Part model, mm, in its own coordinate system. Face numbers are marked on the shaded views. Coordinates: 2 decimals unless noted, no trailing zeros. Order: outer loops, then holes, each group sorted by start corner. A loop starts at its lowest first (then second) coordinate and runs counter-clockwise, first axis right, second up. Notation, with made-up numbers: (68.5, 56) - (120.5, 56) arc R38 ccw to (120.5, 94) - close; hole circle Ø7 at (11.5, 53.5). An arc over 180 degrees is marked (long way). Use a Markdown table: item, result. Add a question column.
1) Drop flat-ended pins along their axis: P1, Ø1.5, axis at x = 94.5, y = 57, coming from the +Z side; P2, Ø3, axis at x = -96.5, z = 127.5, coming from the +Y side; P3, Ø1.5, axis at x = 26, z = 43, coming from the +Y side. Give the stop position or say it passes through.
2) Saw through at B-B on y = 15. Count the separate pieces of the cut face and the enclosed holes in it, then the cut area to 3 significant figures.
3) Wall check: L1, parallel to X at y = -2.5, z = 27.5; L2, parallel to Z at x = -96, y = -2; L3, parallel to Z at x = -96.5, y = -2.05. Give the ranges that are in metal, low to high. Write a range as [from, to].
4) Saw through at A-A on z = 9. List the corners of the cut face in (x, y), then the cut area to 3 significant figures.
5) Two-plate mould, pull along X, no slides. Class the marked faces 1 and 2: +X half, -X half, draft (parallel to the pull), parting line (faces both ways), or undercut.
6) Saw through at C-C on x = 33.5. List the corners of the cut face in (y, z), then the cut area to 3 significant figures.
```python
from build123d import *

# Parameters (mm, degrees)
BOSS_EXTRUDE1_DEPTH      = 160
BOSS_EXTRUDE1_2_DEPTH    = 160
LPATTERN1_COUNT          = 3
LPATTERN1_PITCH          = 55
SKETCH2_W                = 201
SKETCH2_H                = 143
BOSS_EXTRUDE2_DEPTH      = 5
BOSS_EXTRUDE3_DEPTH      = 8
M3_CLEARANCE_HOLE1_D     = 3.4
M3_CLEARANCE_HOLE1_DEPTH = 5


with BuildPart() as part:
    # Sketch1 → Boss-Extrude1 (new body)
    with BuildSketch(Plane(origin=(0, 0, 0), x_dir=(1, 0, 0), z_dir=(0, 1, 0))):
        Polygon((-100.5, 5.5), (-92.5, 5.5), (-92.5, 2.5), (-97.5, 2.5), (-97.5, -2.5), (-92.5, -2.5), (-92.5, -5.5), (-100.5, -5.5), align=None)
    boss_extrude1 = extrude(amount=BOSS_EXTRUDE1_DEPTH)



with BuildPart() as body_2:
    # Sketch1 → Boss-Extrude1 2 (new body)
    with BuildSketch(Plane(origin=(0, 0, 0), x_dir=(1, 0, 0), z_dir=(0, 1, 0))):
        Polygon((100.5, -5.5), (100.5, 5.5), (92.5, 5.5), (92.5, 2.5), (97.5, 2.5), (97.5, -2.5), (92.5, -2.5), (92.5, -5.5), align=None)
    boss_extrude1_2 = extrude(amount=BOSS_EXTRUDE1_2_DEPTH)


with BuildPart() as lpattern1_1:
    # LPattern1: pattern copy
    add(boss_extrude1.moved(Location(Vector(0, 0, 1) * (1 * LPATTERN1_PITCH))))


with BuildPart() as lpattern1_2:
    # LPattern1: pattern copy
    add(boss_extrude1.moved(Location(Vector(0, 0, 1) * (2 * LPATTERN1_PITCH))))


with BuildPart() as lpattern1_3:
    # LPattern1: pattern copy
    add(boss_extrude1_2.moved(Location(Vector(0, 0, 1) * (1 * LPATTERN1_PITCH))))


with BuildPart() as lpattern1_4:
    # LPattern1: pattern copy
    add(boss_extrude1_2.moved(Location(Vector(0, 0, 1) * (2 * LPATTERN1_PITCH))))


with BuildPart() as part_1:
    add(part.part)

    add(body_2.part)  # Boss-Extrude2 merges body 2

    add(lpattern1_1.part)  # Boss-Extrude2 merges LPattern1_1

    add(lpattern1_2.part)  # Boss-Extrude2 merges LPattern1_2

    add(lpattern1_3.part)  # Boss-Extrude2 merges LPattern1_3

    add(lpattern1_4.part)  # Boss-Extrude2 merges LPattern1_4
    # Sketch2 → Boss-Extrude2 (add)
    with BuildSketch(Plane.XZ):
        with Locations((0, 66)):
            Rectangle(SKETCH2_W, SKETCH2_H)
    extrude(amount=BOSS_EXTRUDE2_DEPTH)

    # Sketch3 → Boss-Extrude3 (add)
    with BuildSketch(Plane.ZY.offset(100.5)):
        Polygon((5.5, 160), (13.816526412, 160), (27.5, 101.834227561), (41.183473588, 160), (49.5, 160), (49.5, 151.683473588), (32.636492883, 80), (49.5, 8.316526412), (49.5, 0), (41.183473588, 0), (27.5, 58.165772439), (13.816526412, 0), (5.5, 0), (5.5, 8.316526412), (22.363507117, 80), (5.5, 151.683473588), align=None)
        Polygon((104.5, 151.683473588), (104.5, 160), (96.183473588, 160), (82.5, 101.834227561), (68.816526412, 160), (60.5, 160), (60.5, 151.683473588), (77.363507117, 80), (60.5, 8.316526412), (60.5, 0), (68.816526412, 0), (82.5, 58.165772439), (96.183473588, 0), (104.5, 0), (104.5, 8.316526412), (87.636492883, 80), align=None)
    boss_extrude3 = extrude(amount=-BOSS_EXTRUDE3_DEPTH)

    # Mirror1: Boss-Extrude3 across plane
    add(boss_extrude3.mirror(Plane(origin=(0, 0, 0), x_dir=(0, 0, 1), z_dir=(1, 0, 0))))

    # M3 Clearance Hole1
    with Locations(Plane(origin=(0, 0, 0), x_dir=(1, 0, 0), z_dir=(0, 1, 0))):
        with Locations((-96.5, -27.5), (-96.5, -82.5), (96.5, -82.5), (96.5, -27.5), (-96.5, -127.5), (96.5, -127.5)):
            Hole(M3_CLEARANCE_HOLE1_D / 2, depth=M3_CLEARANCE_HOLE1_DEPTH)


solid = part_1.part
```
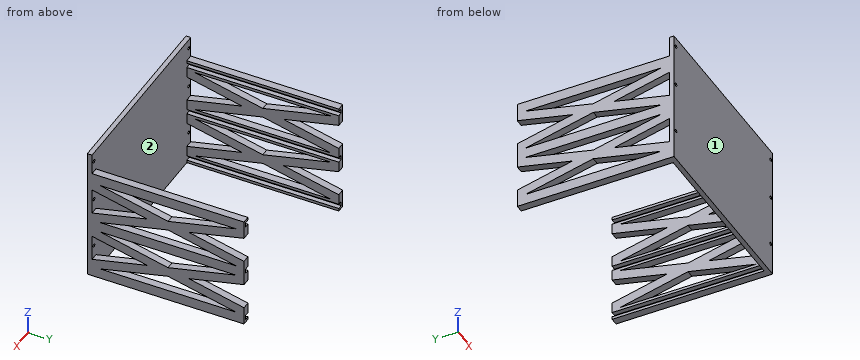
Results are:
| question | item | result |
|---|---|---|
| 1 | P1 | z = 115.5 |
| 1 | P2 | through |
| 1 | P3 | y = 0 |
| 2 | separate pieces | 14 |
| 2 | enclosed holes | 0 |
| 2 | area | 1,040 mm2 |
| 3 | L1 | [-100.5, -98.2], [-94.8, 94.8], [98.2, 100.5] |
| 3 | L2 | [-5.5, 25.88], [29.12, 80.88], [84.12, 125.88], [129.12, 137.5] |
| 3 | L3 | [-5.5, 25.8], [29.2, 80.8], [84.2, 125.8], [129.2, 137.5] |
| 4 | outline | (-100.5, -5) - (100.5, -5) - (100.5, 23.19) - (92.5, 23.19) - (92.5, 0) - (-92.5, 0) - (-92.5, 23.19) - (-100.5, 23.19) - close; (-100.5, 136.81) - (-92.5, 136.81) - (-92.5, 160) - (-100.5, 160) - close; (92.5, 136.81) - (100.5, 136.81) - (100.5, 160) - (92.5, 160) - close |
| 4 | area | 1,750 mm2 |
| 5 | face 1 | draft |
| 5 | face 2 | undercut |
| 6 | outline | (-5, -5.5) - (0, -5.5) - (0, 137.5) - (-5, 137.5) - close |
| 6 | area | 715 mm2 |
